Autodesk Inventor part; units mm, degrees
ref_plane "YZ Plane" through (0, 0, 0) normal (1, 0, 0) x (0, 1, 0)
ref_plane "XZ Plane" through (0, 0, 0) normal (0, 1, 0) x (-1, 0, 0)
ref_plane "XY Plane" through (0, 0, 0) normal (0, 0, 1) x (1, 0, 0)
sketch "Sketch1" plane through (0, 0, 0) normal (0, 1, 0) x (-1, 0, 0)
  line L0 (0, 0) -> (0, -88.9)
  line L1 (0, -88.9) -> (-127, -88.9)
  line L2 (-127, -88.9) -> (-127, 0)
  line L3 (-127, 0) -> (0, 0)
  line L4 (3.175, -92.075) -> (3.175, 3.175)
  line L5 (3.175, 3.175) -> (-130.175, 3.175)
  line L6 (-130.175, 3.175) -> (-130.175, -92.075)
  line L7 (-130.175, -92.075) -> (3.175, -92.075)
  line L8 (0, 0) -> (0, -88.9)
  line L9 (0, -88.9) -> (-40.7416, -88.9)
  line L10 (-40.7416, -88.9) -> (-40.7416, 0)
  line L11 (-40.7416, 0) -> (0, 0)
  line L12 (-40.7416, 0) -> (-40.7416, -88.9)
  line L13 (-40.7416, -88.9) -> (-43.9166, -88.9)
  line L14 (-43.9166, -88.9) -> (-43.9166, 0)
  line L15 (-43.9166, 0) -> (-40.7416, 0)
  line L16 (-127, -88.9) -> (-127, 0)
  line L17 (-127, 0) -> (-86.2584, 0)
  line L18 (-86.2584, 0) -> (-86.2584, -88.9)
  line L19 (-86.2584, -88.9) -> (-127, -88.9)
  line L20 (-86.2584, 0) -> (-86.2584, -88.9)
  line L21 (-86.2584, -88.9) -> (-83.0834, -88.9)
  line L22 (-83.0834, -88.9) -> (-83.0834, 0)
  line L23 (-83.0834, 0) -> (-86.2584, 0)
  dimension "d0" = 88.9
  dimension "d1" = 127
  dimension "d2" = 3.175
  dimension "d3" = 40.7416
  dimension "d4" = 3.175
  dimension "d5" = 40.7416
  dimension "d6" = 3.175
extrude "Extrusion1" add sketch "Sketch1" along normal blind 50.8 contours L10 L1 L14 L3 | L22 L1 L18 L3 | L7 L6 L5 L4
sketch "Sketch2" plane through (0, 0, 0) normal (0, -1, 0) x (1, 0, 0)
  line L0 (-3.175, 3.175) -> (130.175, 3.175)
  line L1 (-3.175, 3.175) -> (130.175, 3.175)
  line L2 (130.175, 3.175) -> (130.175, 0)
  line L3 (130.175, 0) -> (-3.175, 0)
  line L4 (-3.175, 0) -> (-3.175, 3.175)
  point P0 (0, 0)
extrude "Extrusion2" add sketch "Sketch2" along normal blind 2.54
sketch "Sketch3" plane through (0, 0, 0) normal (0, -1, 0) x (1, 0, 0)
  line L0 (130.175, -92.075) -> (-3.175, -92.075)
  line L1 (-3.175, -92.075) -> (130.175, -92.075)
  line L2 (130.175, -92.075) -> (130.175, -88.9)
  line L3 (130.175, -88.9) -> (-3.175, -88.9)
  line L4 (-3.175, -88.9) -> (-3.175, -92.075)
  point P0 (0, 0)
  dimension "d11" = 3.175
extrude "Extrusion3" add sketch "Sketch3" along normal blind 7.62
sketch "Sketch4" plane through (0, -7.62, 0) normal (0, -1, 0) x (1, 0, 0)
  line L0 (130.175, -92.075) -> (-3.175, -92.075)
  line L1 (-3.175, -92.075) -> (130.175, -92.075)
  line L2 (130.175, -92.075) -> (130.175, 3.175)
  line L3 (130.175, 3.175) -> (-3.175, 3.175)
  line L4 (-3.175, 3.175) -> (-3.175, -92.075)
  line L5 (0, 0) -> (127, 0)
  line L6 (127, 0) -> (127, -88.9)
  line L7 (127, -88.9) -> (0, -88.9)
  line L8 (0, -88.9) -> (0, 0)
  point P0 (0, 0)
extrude "Extrusion4" add sketch "Sketch4" against normal blind 3.175
sketch "Sketch9" plane through (-3.175, -7.62, 3.175) normal (0, 0, 1) x (1, 0, 0)
  line L0 (0, 58.42) -> (0, 0) construction
  line L1 (0, 0) -> (0, -12.7) construction
  line L2 (0, -12.7) -> (0, 0) construction
  line L3 (0, -12.7) -> (12.7, -12.7) construction
  line L4 (0, 0) -> (133.35, 0) construction
  line L5 (133.35, 0) -> (133.35, -12.7) construction
  line L6 (133.35, -12.7) -> (120.65, -12.7) construction
  line L7 (0, 0) -> (12.7, -12.7)
  line L8 (12.7, -12.7) -> (120.65, -12.7)
  line L9 (120.65, -12.7) -> (133.35, 0)
  line L10 (0, 0) -> (133.35, 0)
  point P0 (3.175, 7.62)
  dimension "d28" = 12.7
  dimension "d29" = 12.7
  dimension "d30" = 90
  dimension "d31" = 12.7
  dimension "d32" = 12.7
extrude "Extrusion9" add sketch "Sketch9" against normal blind 3.175
sketch "Sketch10" plane through (130.175, 50.8, -92.075) normal (0, 0, -1) x (-1, 0, 0)
  line L0 (133.35, -58.42) -> (0, -58.42)
  line L1 (12.7, -71.12) -> (120.65, -71.12)
  line L2 (133.35, -58.42) -> (120.65, -71.12)
  line L3 (0, -58.42) -> (12.7, -71.12)
  line L4 (120.65, -71.12) -> (12.7, -71.12)
  line L5 (12.7, -71.12) -> (0, -58.42)
  line L6 (0, -58.42) -> (133.35, -58.42)
  point P0 (130.175, -50.8)
extrude "Extrusion10" add sketch "Sketch10" against normal blind 3.175
sketch "Sketch11" plane through (130.175, -7.62, -88.9) normal (0.7071068, -0.7071068, 0) x (-0.7071068, -0.7071068, 0)
  line L0 (0, 3.175) -> (0, 0)
  line L1 (17.9605, 3.175) -> (17.9605, 0)
  line L2 (0, 3.175) -> (17.9605, 3.175)
  line L3 (17.9605, 3.175) -> (17.9605, -92.075)
  line L4 (17.9605, -92.075) -> (0, -92.075)
  line L5 (0, -92.075) -> (0, 3.175)
  point P0 (86.6595, -88.9)
extrude "Extrusion11" add sketch "Sketch11" against normal blind 3.175
sketch "Sketch12" plane through (9.525, -20.32, -88.9) normal (-0.7071068, -0.7071068, 0) x (-0.7071068, 0.7071068, 0)
  line L0 (59.2697, 3.175) -> (17.9605, 3.175)
  line L1 (17.9605, -92.075) -> (0, -92.075)
  line L2 (17.9605, 3.175) -> (17.9605, -92.075)
  line L3 (17.9605, -92.075) -> (0, -92.075)
  line L4 (0, -92.075) -> (0, 3.175)
  line L5 (0, 3.175) -> (17.9605, 3.175)
  point P0 (21.1036, -88.9)
  point P1 (0, -92.075)
extrude "Extrusion12" add sketch "Sketch12" against normal blind 3.175
sketch "Sketch13" plane through (127, 0, -88.9) normal (-1, 0, 0) x (0, 0, 1)
  line L0 (0, 50.8) -> (9.525, 50.8) construction
  line L1 (0, 50.8) -> (88.9, 50.8) construction
  line L2 (9.525, 50.8) -> (9.525, 44.45) construction
  circle A0 centre (9.525, 44.45) radius 2.3876
  line L3 (9.525, 44.45) -> (73.025, 44.45) construction
  circle A1 centre (73.025, 44.45) radius 2.3876
  point P0 (88.9, 0)
  dimension "d46" = 9.525
  dimension "d47" = 6.35
  dimension "d48" = 4.7752
  dimension "d49" = 63.5
  dimension "d50" = 4.7752
extrude "Extrusion13" cut sketch "Sketch13" against normal blind 3.175
sketch "Sketch14" plane through (130.175, 50.8, -92.075) normal (0, 0, -1) x (-1, 0, 0)
  line L0 (0, -53.34) -> (0, 0) construction
  line L1 (0, 0) -> (0, -6.35) construction
  line L2 (0, -6.35) -> (9.5244, -6.2428) construction
  line L3 (9.5244, -6.2428) -> (98.4244, -6.2428) construction
  circle A0 centre (9.5244, -6.2428) radius 2.3876
  circle A1 centre (98.4244, -6.2428) radius 2.3876
  point P0 (130.175, -50.8)
  dimension "d51" = 6.35
  dimension "d52" = 9.525
  dimension "d53" = 88.9
  dimension "d54" = 4.7752
  dimension "d55" = 4.7752
extrude "Extrusion14" cut sketch "Sketch14" against normal blind 3.175
sketch "Sketch15" plane through (9.525, -20.32, -92.075) normal (0, -1, 0) x (1, 0, 0)
  line L0 (120.65, 0) -> (107.95, 0)
  line L1 (0, 3.175) -> (107.95, 3.175)
  line L2 (107.95, 0) -> (0, 0)
  line L3 (0, 0) -> (0, 3.175)
  line L4 (0, 3.175) -> (107.95, 3.175)
  line L5 (107.95, 3.175) -> (107.95, 0)
  point P0 (-9.525, 92.075)
extrude "Extrusion15" add sketch "Sketch15" along normal blind 29.21
sketch "Sketch16" plane through (9.525, -49.53, -92.075) normal (-1, 0, 0) x (0, 0, 1)
  line L0 (0, 29.21) -> (0, 0)
  line L1 (0, 0) -> (38.1, 0)
  line L2 (38.1, 0) -> (0, 29.21)
  line L3 (3.175, 22.7751) -> (3.175, 3.175)
  line L4 (3.175, 3.175) -> (28.7404, 3.175)
  line L5 (28.7404, 3.175) -> (3.175, 22.7751)
  point P0 (92.075, 49.53)
  dimension "d60" = 38.1
  dimension "d61" = 3.175
extrude "Extrusion16" add sketch "Sketch16" against normal blind 107.95
properties part number "BeadCompartments_5"
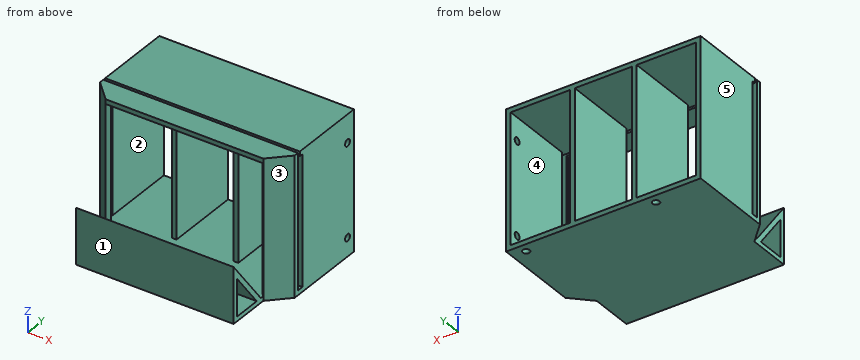
Part model, mm, in its own coordinate system. Face numbers are marked on the shaded views. A direction names the side the tool comes from. Coordinates: 2 decimals unless noted, no trailing zeros. Order: outer loops, then holes, each group sorted by start corner. A loop starts at its lowest first (then second) coordinate and runs counter-clockwise, first axis right, second up.
(1) Slice it at A-A, the plane x = 72.5. Write the cut outline in (y, z) (3 decimals).
Check sheet entries:
outline: (-49.53, -92.075) - (50.8, -92.075) - (50.8, -88.9) - (-22.754, -88.9) - (-49.53, -53.975) - close; (-20.32, 0) - (-4.445, 0) - (-4.445, 3.175) - (-20.32, 3.175) - close; (-2.54, 0) - (50.8, 0) - (50.8, 3.175) - (-2.54, 3.175) - close; hole (-46.355, -88.9) - (-26.755, -88.9) - (-46.355, -63.335) - close
(2) Pin check, flat tips, straight feed: pin 1 Ø2.5 at (x, z) = (128.5, -54.5) entering from -Y (3 decimals); pin 2 Ø20.5 at (x, z) = (64, -75.5) entering from +Y; pin 3 Ø6 at (x, y) = (72, -38) entering from +Z. Stop position of each tip, or through.
Check sheet entries:
pin 1: stops at y = -10.545
pin 2: stops at y = -25.17
pin 3: stops at z = -65.1
(3) Probe L1, parallel to X at y = 40.5, z = -27.5 (3 decimals); L2, parallel to Z at x = 18, y = 6.5 (3 decimals); L3, parallel to Y at x = 42, z = -18.5. List the from-to ranges inside material, lowest first.
Check sheet entries:
L1: x = -3.175 to 0, 40.742 to 43.917, 83.083 to 86.258, 127 to 130.175
L2: z = -92.075 to -88.9, 0 to 3.175
L3: y = 0 to 50.8
(4) Pull direction X, two halves, no side cores. Call the marked faces 1, 2 and 3: pulls with the +X half, pulls with the -X half, needs draft (parallel to the pull), parting line crosses it, or undercut.
Check sheet entries:
face 1: needs draft
face 2: undercut
face 3: pulls with the +X half
(5) Slice it at C-C, the plane z = -31. Write the cut outline in (x, y) (3 decimals), and give its area (3 significant figures).
Check sheet entries:
outline: (-3.175, -7.62) - (9.525, -20.32) - (11.77, -18.075) - (0, -6.305) - (0, -4.445) - (-3.175, -4.445) - close; (-3.175, 0) - (0, 0) - (0, 50.8) - (-3.175, 50.8) - close; (40.742, 0) - (43.917, 0) - (43.917, 50.8) - (40.742, 50.8) - close; (83.083, 0) - (86.258, 0) - (86.258, 50.8) - (83.083, 50.8) - close; (115.23, -18.075) - (117.475, -20.32) - (130.175, -7.62) - (130.175, -4.445) - (127, -4.445) - (127, -6.305) - close; (127, 0) - (130.175, 0) - (130.175, 50.8) - (127, 50.8) - close
area: 771 mm2
(6) Tool access for the marked faces 4 and 5: list every direction of +Z, -Z, +X, -X, +Y, -Y with a clear straight run to the whole face (end or side of a thin tool).
Check sheet entries:
face 4: +Y
face 5: +Z, -Z, -X, +Y, -Y
(7) Slice it at B-B, the plane y = 16. Write the cut outline in (x, z) (3 decimals), and give its area (3 significant figures).
Check sheet entries:
outline: (-3.175, -92.075) - (130.175, -92.075) - (130.175, 3.175) - (-3.175, 3.175) - close; hole (0, -88.9) - (40.742, -88.9) - (40.742, 0) - (0, 0) - close; hole (43.917, -88.9) - (83.083, -88.9) - (83.083, 0) - (43.917, 0) - close; hole (86.258, -88.9) - (127, -88.9) - (127, 0) - (86.258, 0) - close
area: 1,980 mm2
(8) Slice it at D-D, the plane y = -32. Write the cut outline in (x, z) (3 decimals), and give its area (3 significant figures).
Check sheet entries:
outline: (9.525, -92.075) - (117.475, -92.075) - (117.475, -88.9) - (9.525, -88.9) - close; (9.525, -82.059) - (117.475, -82.059) - (117.475, -76.84) - (9.525, -76.84) - close
area: 906 mm2
